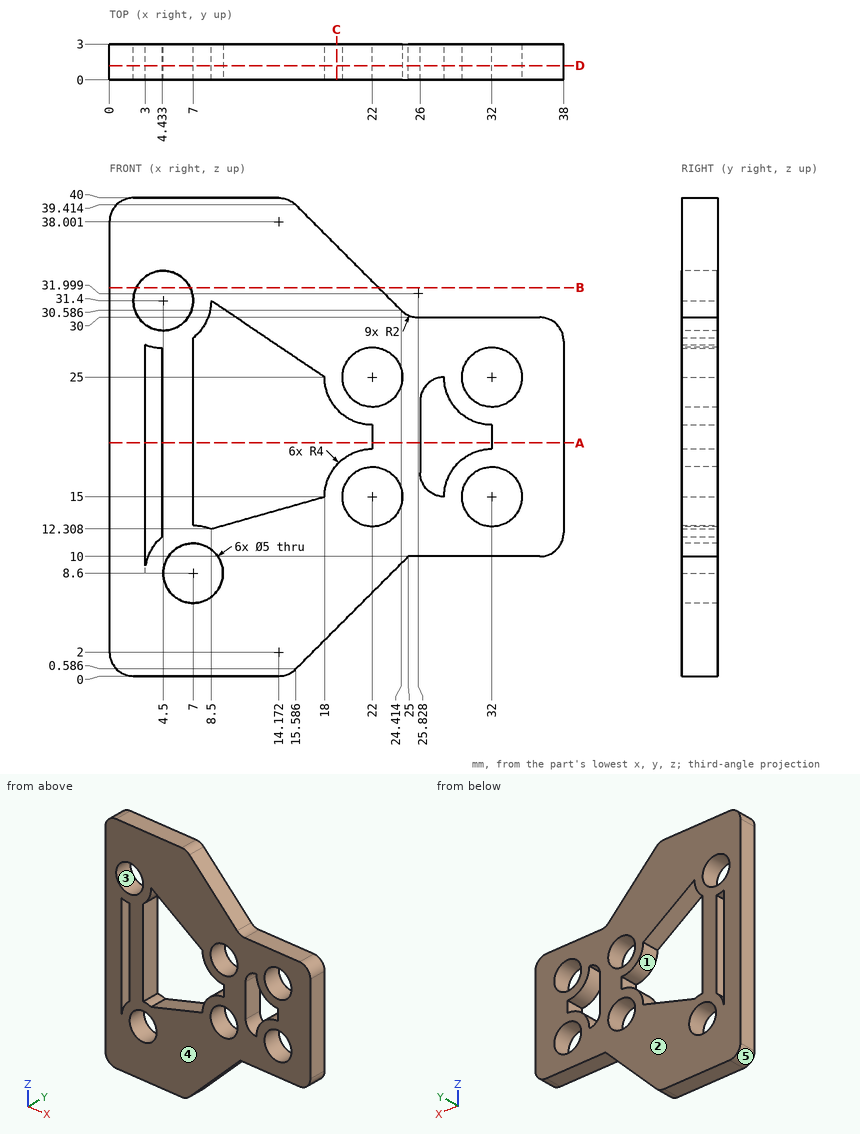
Design review of the part shown in the three views and the two pictorial views. Dimensions are in mm from the part's minimum x, y and z. A direction names the side the tool comes from. Give positions to 0.01 mm unless a question says otherwise; leave off trailing zeros. Write each loop counter-clockwise with the first axis right and the second up, starting at its lowest first coordinate (ties: lowest second). Pieces come first, ordered by that corner, then holes.
(1) Mouldability with a two-part tool opening along Z and no side actions: class the marked faces 3, 4 and 5 as +Z half, -Z half, draft (parallel to the pull), parting line (faces both ways), or undercut.
Checked values:
face 3: undercut
face 4: draft
face 5: -Z half
(2) Add section B-B (z = 32.5). Give the boundary of the cut face in (x, y) (1 decimal).
Checked values:
outline: (0, 0) - (2.3, 0) - (2.3, 3) - (0, 3) - close; (6.7, 0) - (22.5, 0) - (22.5, 3) - (6.7, 3) - close
(3) Wall thickness on line 1 along Z through (x, y) = (33, 0.45); line 2 along X through (y, z) = (1.35, 38); line 3 along Z through (x, y) = (28.5, 1.65) (1 decimal): over which ranges is each line inside the solid? List them lowest first.
Checked values:
line 1: z = 10 to 12.71, 17.29 to 22.71, 27.29 to 30
line 2: x = 0 to 17
line 3: z = 10 to 16.9, 23.1 to 30
(4) Clearance check with flat-ended pins moving along their axes: pin 1 Ø4.5 at (x, z) = (22, 25) entering from +Y; pin 2 Ø1 at (x, y) = (29.5, 1) entering from +Z. State where each tip first meets the part, or that it passes through.
Checked values:
pin 1: passes through
pin 2: stops at z = 30
(5) Tool access review of the marked faces 1 and 2: name each direction out of +Z, -Z, +X, -X, +Y, -Y from which nothing blocks a thin tool from reaching the whole face with its end or side.
Checked values:
face 1: +Y, -Y
face 2: +Z, -Z, +X, -X, +Y
(6) Add section D-D (y = 1.2). Give the number of separate pieces and of enclosed holes in the cut face.
Checked values:
separate pieces: 1
enclosed holes: 9
(7) Add section C-C (x = 19). Give the boundary of the cut face in (y, z) (1 decimal).
Checked values:
outline: (0, 4) - (3, 4) - (3, 17.6) - (0, 17.6) - close; (0, 22.4) - (3, 22.4) - (3, 36) - (0, 36) - close
(8) Add section A-A (z = 19.5). Give the boundary of the cut face in (x, y).
Checked values:
outline: (0, 0) - (3, 0) - (3, 3) - (0, 3) - close; (4.43, 0) - (7, 0) - (7, 3) - (4.43, 3) - close; (22, 0) - (26, 0) - (26, 3) - (22, 3) - close; (32, 0) - (38, 0) - (38, 3) - (32, 3) - close
